Input: part model. Units: mm. Frame: model coordinates. Coordinates: 2 decimals unless noted, no trailing zeros. Write each loop counter-clockwise with the first axis right and the second up, starting at its lowest first coordinate (ties: lowest second). Pieces come first, ordered by that corner, then holes. Notation, with made-up numbers: (79, 11) - (120, 11) arc R28 cw to (120, 43) - close; hole circle Ø8 at (15, 65). An arc over 180 degrees is marked (long way). Use CSV: the item, a comma, the result in double quotes.
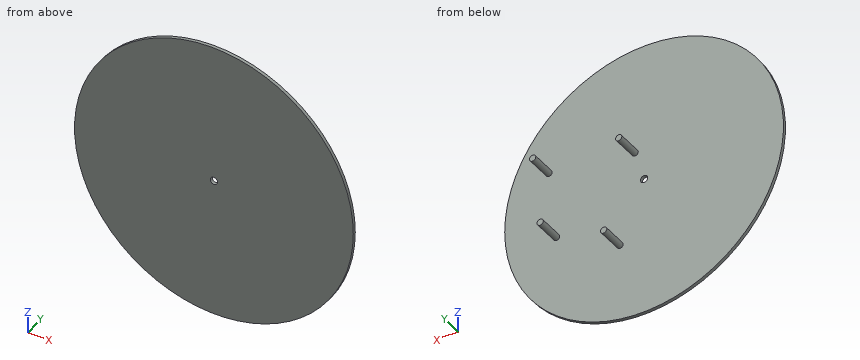
```python
from build123d import *

# Parameters (mm, degrees)
SKETCH1_R            = 111.264222233
SKETCH1_R_2          = 2.92
SKETCH1_R_3          = 2.5
BOSS_EXTRUDE12_DEPTH = 2.5
SKETCH5_R            = 2.5
BOSS_EXTRUDE15_DEPTH = 23
SKETCH6_R            = 2.5
BOSS_EXTRUDE16_DEPTH = 23
SKETCH7_R            = 2.5
BOSS_EXTRUDE17_DEPTH = 23
SKETCH3_R            = 2.5
BOSS_EXTRUDE18_DEPTH = 23


with BuildPart() as part:
    # Sketch1 → Boss-Extrude12 (new body)
    with BuildSketch(Plane(origin=(0, 0, 0), x_dir=(1, 0, 0), z_dir=(0, 1, 0))):
        Circle(SKETCH1_R)
        Circle(SKETCH1_R_2, mode=Mode.SUBTRACT)
        with Locations((75.852459016, -35)):
            Circle(SKETCH1_R_3, mode=Mode.SUBTRACT)
        with Locations((69.852459016, 21)):
            Circle(SKETCH1_R_3, mode=Mode.SUBTRACT)
        with Locations((19.152459016, 47.9)):
            Circle(SKETCH1_R_3, mode=Mode.SUBTRACT)
        with Locations((7.152459016, -24.6)):
            Circle(SKETCH1_R_3, mode=Mode.SUBTRACT)
    extrude(amount=BOSS_EXTRUDE12_DEPTH)

    # Sketch5 → Boss-Extrude15 (add)
    with BuildSketch(Plane(origin=(0, 0, 0), x_dir=(-1, 0, 0), z_dir=(0, -1, 0))):
        with Locations((-19.152459016, 47.9)):
            Circle(SKETCH5_R)
    extrude(amount=-BOSS_EXTRUDE15_DEPTH)

    # Sketch6 → Boss-Extrude16 (add)
    with BuildSketch(Plane(origin=(0, 0, 0), x_dir=(-1, 0, 0), z_dir=(0, -1, 0))):
        with Locations((-69.852459016, 21)):
            Circle(SKETCH6_R)
    extrude(amount=-BOSS_EXTRUDE16_DEPTH)

    # Sketch7 → Boss-Extrude17 (add)
    with BuildSketch(Plane(origin=(0, 0, 0), x_dir=(-1, 0, 0), z_dir=(0, -1, 0))):
        with Locations((-75.852459016, -35)):
            Circle(SKETCH7_R)
    extrude(amount=-BOSS_EXTRUDE17_DEPTH)

    # Sketch3 → Boss-Extrude18 (add)
    with BuildSketch(Plane(origin=(0, 0, 0), x_dir=(-1, 0, 0), z_dir=(0, -1, 0))):
        with Locations((-7.152459016, -24.6)):
            Circle(SKETCH3_R)
    extrude(amount=-BOSS_EXTRUDE18_DEPTH)


solid = part.part
```
(1) Cut plane D-D on x = -54.5. Return loops of the section in (y, z), and give its area (3 significant figures).
Check values:
outline,"(0, -97) - (2.5, -97) - (2.5, 97) - (0, 97) - close"
area,"485 mm^2"
(2) Cut plane C-C on z = 79.5. Return loops of the section in (x, y), and give its area (3 significant figures).
Check values:
outline,"(-77.84, 0) - (77.84, 0) - (77.84, 2.5) - (-77.84, 2.5) - close"
area,"389 mm^2"
(3) Ray query, probe 1 along X at (y, z) = (0.65, 0); probe 2 along Y at (x, z) = (4, -19). Return the intervals inside material, ascending. Write a range as from..to.
Check values:
probe 1,"-111.26..-2.92, 2.92..111.26"
probe 2,"0..2.5"
(4) Cut plane A-A on x = 0. Return loops of the section in (y, z), and give its area (3 significant figures).
Check values:
outline,"(0, -111.26) - (2.5, -111.26) - (2.5, -2.92) - (0, -2.92) - close; (0, 2.92) - (2.5, 2.92) - (2.5, 111.26) - (0, 111.26) - close"
area,"542 mm^2"
(5) Cut plane B-B on y = 14. Return loops of the section in (x, z), and give its area (3 significant figures).
Check values:
outline,"circle Ø5 at (7.15, 24.6); circle Ø5 at (19.15, -47.9); circle Ø5 at (69.85, -21); circle Ø5 at (75.85, 35)"
area,"78.5 mm^2"
(6) Pin query (flat end, axial travel): pin 1 Ø5 at (y, z) = (4.5, 36.5) entering from -X; pin 2 Ø6 at (x, z) = (-53.5, -25) entering from -Y; pin 3 Ø4 at (x, z) = (-40.5, 33) entering from +Y; pin 4 Ø5.5 at (x, z) = (0, 0) entering from +Y. Return the tip coordinate at first contact, or that it passes through.
Check values:
pin 1,"x = -105.62"
pin 2,"y = 0"
pin 3,"y = 2.5"
pin 4,"through"
